```python
from build123d import *

# Parameters (mm, degrees)
SKETCH_1_W          = 14.9
SKETCH_1_H          = 11.5
EXTRUDE_1_DEPTH     = 5.75
SKETCH_2_W          = 0.64
SKETCH_2_H          = 0.64
EXTRUDE_2_DEPTH     = 3.4
CUT_EXTRUDE_1_DEPTH = 21.928031441
SKETCH_4_W          = 12.9
SKETCH_4_H          = 3.75
CUT_EXTRUDE_2_DEPTH = 5


with BuildPart() as part:
    # Эскиз1 → Бобышка-Вытянуть1 (new body)
    with BuildSketch(Plane.XY):
        with Locations((7.45, 5.75)):
            Rectangle(SKETCH_1_W, SKETCH_1_H)
    extrude(amount=EXTRUDE_1_DEPTH)

    # Эскиз2 → Бобышка-Вытянуть2 (add)
    with BuildSketch(Plane.XY.offset(5.75)):
        with Locations((4.95, 2.3)):
            Rectangle(SKETCH_2_W, SKETCH_2_H)
        with Locations((2.45, 2.3)):
            Rectangle(SKETCH_2_W, SKETCH_2_H)
        with Locations((7.45, 2.3)):
            Rectangle(SKETCH_2_W, SKETCH_2_H)
        with Locations((9.95, 2.3)):
            Rectangle(SKETCH_2_W, SKETCH_2_H)
        with Locations((12.45, 2.3)):
            Rectangle(SKETCH_2_W, SKETCH_2_H)
    extrude(amount=EXTRUDE_2_DEPTH)

    # Эскиз3 → Вырез-Вытянуть1 (cut, through all)
    with BuildSketch(Plane.ZY):
        Polygon((0, 0), (0, 3.523806865), (2.536361598, 2.431096681), (3.433362495, 0), align=None)
    extrude(amount=-CUT_EXTRUDE_1_DEPTH, mode=Mode.SUBTRACT)

    # Эскиз4 → Вырез-Вытянуть2 (cut)
    with BuildSketch(Plane(origin=(0, 11.5, 0), x_dir=(1, 0, 0), z_dir=(0, 1, 0))):
        with Locations((7.45, -2.875)):
            Rectangle(SKETCH_4_W, SKETCH_4_H)
    extrude(amount=-CUT_EXTRUDE_2_DEPTH, mode=Mode.SUBTRACT)


solid = part.part
```
CAD build for the part. Positions are in the model's coordinates, mm. A direction names the side the tool comes from. Coordinates: 2 decimals unless noted, no trailing zeros. Order: outer loops, then holes, each group sorted by start corner. A loop starts at its lowest first (then second) coordinate and runs counter-clockwise, first axis right, second up. Notation, with made-up numbers: (77, -39.5) -> (118, -39.5) arc R16 cw to (118, -18.5) -> close; hole circle Ø1 at (7, -18). An arc over 180 degrees is marked (long way). Use one line per item in the form item = value. Start each with the question number.
1) Band-saw the part on D-D on z = 4. Give the cut face in (x, y).
2) Drill centre lines: L1, parallel to Z at x = 2.5, y = 11; L2, parallel to X at y = 10.75, z = 3.5; L3, parallel to Z at x = 5.25, y = 5. Where is each one in solid material? Low to high. Write a range as [from, to].
3) Band-saw the part on A-A on y = 10.75. Give the cut face in (x, z), then the cut area to 3 significant figures.
4) Pull direction Z, two halves, no side cores. Call faces 3 (the flat face through (7, 9, 4.75)), 4 (the flat face through (7.35, 1.23, 2.98)), 5 (the flat face through (14.9, 7, 3)): +Z half, -Z half, draft (parallel to the pull), parting line (faces both ways), or undercut.
5) Band-saw the part on B-B on z = 7. Give the cut face in (x, y).
6) Tool access for faces 1 (the flat face through (0, 7, 3)), 2 (the flat face through (1, 9, 3)): list every direction of +Z, -Z, +X, -X, +Y, -Y with a clear straight run to the whole face (end or side of a thin tool).
7) Band-saw the part on C-C on x = 5. Give the cut face in (y, z), then the cut area to 3 significant figures.
8) Drop flat-ended pins along their axis: pin 1 (0.7 mm diameter, centred on y = 2, z = 8, fed in from -X); pin 2 (0.7 mm diameter, centred on x = 10, z = 7.5, fed in from -Y); pin 3 (5.5 mm diameter, centred on x = 8.5, y = 8.5, fed in from +Z); pin 4 (1.5 mm diameter, centred on y = 7.5, z = 7, fed in from +X). Give the stop position or say it passes through.
Entries:
q1.outline = (0, 0) -> (14.9, 0) -> (14.9, 11.5) -> (13.9, 11.5) -> (13.9, 6.5) -> (1, 6.5) -> (1, 11.5) -> (0, 11.5) -> close
q2.L1 = [0, 1], [4.75, 5.75]
q2.L2 = [0, 1], [13.9, 14.9]
q2.L3 = [0, 5.75]
q3.outline = (0, 0) -> (14.9, 0) -> (14.9, 5.75) -> (0, 5.75) -> close; hole (1, 1) -> (13.9, 1) -> (13.9, 4.75) -> (1, 4.75) -> close
q3.area = 37.3 mm2
q4.face_3 = undercut
q4.face_4 = -Z half
q4.face_5 = draft
q5.outline = (2.13, 1.98) -> (2.77, 1.98) -> (2.77, 2.62) -> (2.13, 2.62) -> close; (4.63, 1.98) -> (5.27, 1.98) -> (5.27, 2.62) -> (4.63, 2.62) -> close; (7.13, 1.98) -> (7.77, 1.98) -> (7.77, 2.62) -> (7.13, 2.62) -> close; (9.63, 1.98) -> (10.27, 1.98) -> (10.27, 2.62) -> (9.63, 2.62) -> close; (12.13, 1.98) -> (12.77, 1.98) -> (12.77, 2.62) -> (12.13, 2.62) -> close
q6.face_1 = +Z, -Z, -X, +Y, -Y
q6.face_2 = +Y
q7.outline = (0, 3.43) -> (2.43, 2.54) -> (3.52, 0) -> (11.5, 0) -> (11.5, 1) -> (6.5, 1) -> (6.5, 4.75) -> (11.5, 4.75) -> (11.5, 5.75) -> (2.62, 5.75) -> (2.62, 9.15) -> (1.98, 9.15) -> (1.98, 5.75) -> (0, 5.75) -> close
q7.area = 40.9 mm2
q8.pin_1 = 2.13
q8.pin_2 = 1.98
q8.pin_3 = 5.75
q8.pin_4 = through
